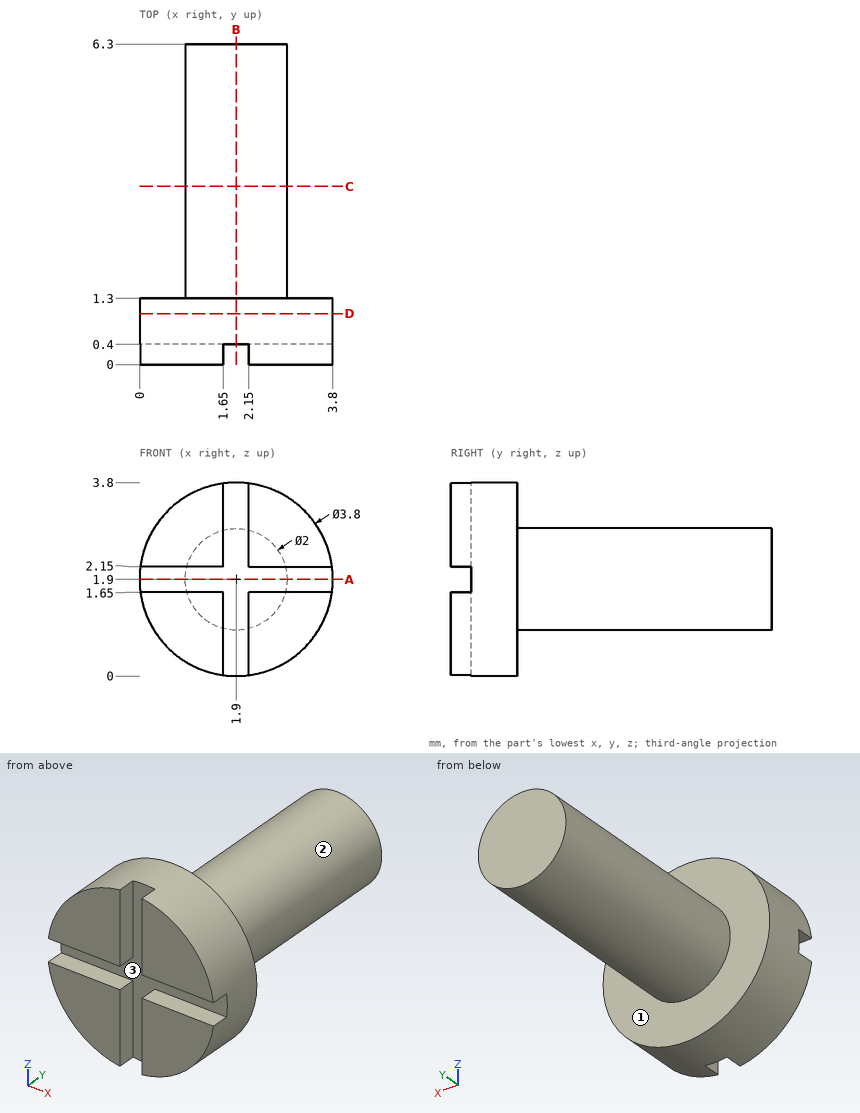
Print and shaded views of the part. All mm, measured from the part's lowest x, y and z. Give positions to 0.01 mm unless a question says otherwise; leave off trailing zeros. Loops run counter-clockwise (first coordinate to the right, second up) from the corner with the lowest first, then second, coordinate; pieces in that order, holes last.
1) Saw through at B-B (x = 1.9). Write the cut outline in (y, z).
2) Pull direction X, two halves, no side cores. Call the marked faces 1, 2 and 3: +X half, -X half, draft (parallel to the pull), parting line (faces both ways), or undercut.
3) Saw through at C-C (y = 3.5). Write the cut outline in (x, z).
4) Wall check: line 1 (Y direction, x = 0.2, z = 2.5); line 2 (Y direction, x = 1.7, z = 1.8); line 3 (X direction, y = 5.25, z = 2.6). Give the ranges that are in metal, low to high.
5) Saw through at D-D (y = 1). Write the cut outline in (x, z), plus the area to 3 significant figures.
6) Saw through at A-A (z = 1.9). Write the cut outline in (x, y), plus the area to 3 significant figures.
Answer block:
1. outline: (0.4, 0) - (1.3, 0) - (1.3, 0.9) - (6.3, 0.9) - (6.3, 2.9) - (1.3, 2.9) - (1.3, 3.8) - (0.4, 3.8) - close
2. face 1: draft
2. face 2: parting line
2. face 3: undercut
3. outline: circle Ø2 at (1.9, 1.9)
4. line 1: y = 0 to 1.3
4. line 2: y = 0.4 to 6.3
4. line 3: x = 1.19 to 2.61
5. outline: circle Ø3.8 at (1.9, 1.9)
5. area: 11.3 mm2
6. outline: (0, 0.4) - (3.8, 0.4) - (3.8, 1.3) - (2.9, 1.3) - (2.9, 6.3) - (0.9, 6.3) - (0.9, 1.3) - (0, 1.3) - close
6. area: 13.4 mm2
